Input: part model. Units: mm. Frame: model coordinates. A direction names the side the tool comes from. Give positions to 0.01 mm unless a question says otherwise; leave off trailing zeros. Order: outer loops, then holes, each group sorted by start corner. A loop starts at its lowest first (then second) coordinate and runs counter-clockwise, first axis right, second up. Notation, with made-up numbers: (78.5, 76) - (124.5, 76) arc R15 cw to (124.5, 105) - close; hole circle Ø2 at (17.25, -21.5). An arc over 180 degrees is marked (long way). Answer in a Markdown table with one row per item. Add a question column.
1. Section query C-C on z = -7.25. Return loops of the section in (x, y), and give its area (3 significant figures).
2. Contact query for flat-ended pins moving along their axis: pin 1 (4 mm diameter, centred on y = -35.5, z = 1, fed in from +X); pin 2 (0.9 mm diameter, centred on x = 28.5, y = -1.5, fed in from +Z); pin 3 (1.9 mm diameter, centred on x = 27.5, y = -18, fed in from -Z). Output: stop coordinate, or through.
3. Section query D-D on x = 3. Return loops of the section in (y, z), and give its area (3 significant figures).
4. Ray query, line 1 (X direction, y = -1, z = -1.75); line 2 (Z direction, x = 5, y = -18); line 3 (Y direction, x = 6.5, z = 1.25). Return the intervals inside material, ascending. Write a range as [from, to].
5. Section query A-A on x = 18.5. Return loops of the section in (y, z).
6. Section query B-B on y = -27.5. Return loops of the section in (x, z), and give its area (3 significant figures).
7. Access query for faces 1 (the face through (29, -2, 9.056)), 2 (the face through (1.53, -46.1, 4.74)), 3 (the face through (23.87, -46.1, 4.74)). Directions: +Z, -Z, +X, -X, +Y, -Y. A direction counts if a zero-diameter tool reaches every point of the face in a straight line with its end or side. Return the directions, or none.
```python
from build123d import *

# Parameters (mm, degrees)
F1_DEPTH   = 25.4
F2_R       = 5.08
F1_FACE_W  = 15.24
F1_FACE_H  = 30.1367967168
F1_FACE1_W = 15.24
F1_FACE1_H = 10.5165233221
F5_DEPTH   = 6.35


with BuildPart() as f1:
    # F0 (on Right) → F1 (new body)
    with BuildSketch(Plane.YZ):
        Polygon((-56.3605315983, 6.1871875077), (-56.3605315983, -9.6700796857), (4.7612222843, -9.6700796857), (4.7612222843, 6.1871875077), (4.7612222843, 14.1358673573), (-33.5322959741, 14.1358673573), (-37.6872867346, 6.1871875077), align=None)
    extrude(amount=F1_DEPTH)

    # F2
    f2_edges = [f1.edges().sort_by_distance(p)[0] for p in [
        (25.4, -56.360532, -1.741446),
        (12.7, -56.360532, 6.187188),
        (0, -56.360532, -1.741446),
        (25.4, -47.023909, 6.187188),
        (25.4, -35.609791, 10.161527),
        (12.7, -33.532296, 14.135867),
        (12.7, -37.687287, 6.187188),
        (25.4, -14.385537, 14.135867),
        (0, -14.385537, 14.135867),
        (12.7, 4.761222, 14.135867),
        (25.4, 4.761222, 2.232894),
        (25.4, -25.799655, -9.67008),
        (0, 4.761222, 2.232894),
        (0, -25.799655, -9.67008),
        (0, -35.609791, 10.161527),
        (0, -47.023909, 6.187188),
    ]]
    fillet(f2_edges, radius=F2_R)

    # F1_face (on face) → F3 section 0
    with BuildSketch(Plane(origin=(12.7, -15.3871760741, 14.1358673573), x_dir=(1, 0, 0), z_dir=(0, 0, 1))):
        Rectangle(F1_FACE_W, F1_FACE_H)
    # F1_face1 (on face) → F3 section 1
    with BuildSketch(Plane(origin=(12.7, -46.0222699373, 6.1871875077), x_dir=(1, 0, 0), z_dir=(0, 0, 1))):
        Rectangle(F1_FACE1_W, F1_FACE1_H)
    loft()

    # F4 (on face) → F5 (join)
    with BuildSketch(Plane.YZ.offset(25.4)):
        with BuildLine():
            Line((-0.3187777157, 9.0558673573), (-3.2266356666, 9.0558673573))
            add(Edge.make_bspline(
                [(-3.2266356666, 9.0558673573), (-10.6613118154, 6.5028903713), (-21.8331213212, -4.5900796857)],
                knots=[0.4644506535, 0.4644506535, 0.4644506535, 1.8030216535, 1.8030216535, 1.8030216535], degree=2, weights=[1, 0.7842651602, 1]))
            Line((-21.8331213212, -4.5900796857), (-9.1981538469, -4.5900796857))
            add(Edge.make_bspline(
                [(-9.1981538469, -4.5900796857), (-1.8305878019, 2.7254934529), (-0.3187777157, 6.9107739232)],
                knots=[4.9446143071, 4.9446143071, 4.9446143071, 5.9063398106, 5.9063398106, 5.9063398106], degree=2, weights=[1, 0.8865961919, 1]))
            Line((-0.3187777157, 6.9107739232), (-0.3187777157, 9.0558673573))
        make_face()
    extrude(amount=F5_DEPTH)


solid = f1.part
```
Answer:
| question | item | result |
|---|---|---|
| 1 | outline | (0.75, -53.94) arc R5.08 ccw to (5.08, -56.36) - (20.32, -56.36) arc R5.08 ccw to (24.65, -53.94) - (24.65, 2.34) arc R5.08 ccw to (20.32, 4.76) - (5.08, 4.76) arc R5.08 ccw to (0.75, 2.34) - close |
| 1 | area | 1,450 mm² |
| 2 | pin 1 | stops at x = 25.4 |
| 2 | pin 2 | stops at z = 9.06 |
| 2 | pin 3 | stops at z = -4.59 |
| 3 | outline | (-55.92, -9.22) - (4.32, -9.22) - (4.32, 9.06) arc R4.63 ccw to (-0.32, 13.69) - (-30.46, 13.69) arc R4.63 ccw to (-34.56, 11.2) - (-35.87, 8.71) arc R5.53 cw to (-40.76, 5.74) - (-51.28, 5.74) arc R4.63 ccw to (-55.92, 1.11) - close |
| 3 | area | 1,210 mm² |
| 4 | line 1 | x = [0, 25.4] |
| 4 | line 2 | z = [-9.67, 14.14] |
| 4 | line 3 | y = [-56.36, 4.76] |
| 5 | outline | (-56.36, -9.67) - (4.76, -9.67) - (4.76, 9.06) arc R5.08 ccw to (-0.32, 14.14) - (-30.46, 14.14) arc R5.08 ccw to (-33.84, 12.84) - (-51.28, 6.19) arc R5.08 ccw to (-56.36, 1.11) - close; hole (-40.76, 6.19) arc R5.08 ccw to (-38.84, 6.57) - close |
| 6 | outline | (0, -4.59) arc R5.08 ccw to (5.08, -9.67) - (20.32, -9.67) arc R5.08 ccw to (25.4, -4.59) - (25.4, 9.06) arc R5.08 ccw to (20.32, 14.14) - (5.08, 14.14) arc R5.08 ccw to (0, 9.06) - close |
| 6 | area | 583 mm² |
| 7 | face 1 | +Z, +X, +Y, -Y |
| 7 | face 2 | +Z, -X, -Y |
| 7 | face 3 | +Z, +X, -Y |
